For this review, take the finished solid that the model builds, in its own axes (mm). Face numbers are marked on the shaded views. Coordinates: 2 decimals unless noted, no trailing zeros. Loops run counter-clockwise (first coordinate to the right, second up) from the corner with the lowest first, then second, coordinate; pieces in that order, holes last. Notation, with made-up numbers: M 58,56 L 108,56 A16 cw 108,85 Z; hole C 73,63 d5. An arc over 180 degrees is marked long. Put each result on its own line as item: value.
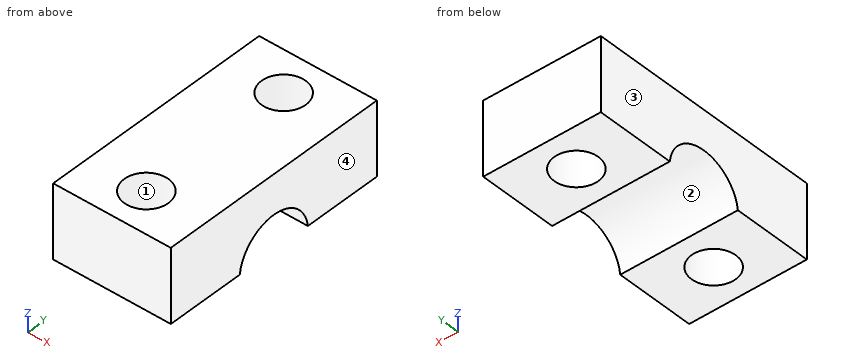
```python
from build123d import *

# Parameters (mm, degrees)
BOSS_EXTRUDE1_DEPTH = 12
SKETCH2_R           = 2.25
CUT_EXTRUDE1_DEPTH  = 19.761663039
SKETCH3_W           = 12
SKETCH3_H           = 24
CUT_EXTRUDE2_DEPTH  = 0.5


with BuildPart() as part:
    # Sketch1 → Boss-Extrude1 (new body)
    with BuildSketch(Plane(origin=(0, 0, 0), x_dir=(0, 0, -1), z_dir=(1, 0, 0))):
        with BuildLine():
            Line((8, -4), (8, -12))
            Line((8, -12), (0, -12))
            Line((0, -12), (0, 12))
            Line((0, 12), (8, 12))
            Line((8, 12), (8, 4))
            ThreePointArc((8, 4), (4, 0), (8, -4))
        make_face()
    extrude(amount=BOSS_EXTRUDE1_DEPTH)

    # Sketch2 → Cut-Extrude1 (cut, through all)
    with BuildSketch(Plane.XY):
        with Locations((6, 8)):
            Circle(SKETCH2_R)
        with Locations((6, -8)):
            Circle(SKETCH2_R)
    extrude(amount=-CUT_EXTRUDE1_DEPTH, mode=Mode.SUBTRACT)

    # Sketch3 → Cut-Extrude2 (cut)
    with BuildSketch(Plane(origin=(0, 0, -8), x_dir=(-1, 0, 0), z_dir=(0, 0, -1))):
        with Locations((-6, 0)):
            Rectangle(SKETCH3_W, SKETCH3_H)
    extrude(amount=-CUT_EXTRUDE2_DEPTH, mode=Mode.SUBTRACT)


solid = part.part
```
(1) Add section A-A (y = 8). Write out the cut boundary in (x, z), plus the area to 4 significant figures.
Determined:
outline: M 0,-7.5 L 3.75,-7.5 L 3.75,0 L 0,0 Z; M 8.25,-7.5 L 12,-7.5 L 12,0 L 8.25,0 Z
area: 56.25 mm^2
(2) Draft analysis for pull direction X (two halves, no side actions). For the marked faces 1, 2, 3 and 4, state which applies: +X half, -X half, draft (parallel to the pull), parting line (faces both ways), or undercut.
Determined:
face 1: undercut
face 2: draft
face 3: -X half
face 4: +X half
(3) Add section B-B (z = -6). Write out the cut boundary in (x, y), plus the area to 3 significant figures.
Determined:
outline: M 0,-12 L 12,-12 L 12,-3.46 L 0,-3.46 Z; M 0,3.46 L 12,3.46 L 12,12 L 0,12 Z; hole C 6,-8 d4.5; hole C 6,8 d4.5
area: 173 mm^2
(4) Add section D-D (z = -1.5). Write out the cut boundary in (x, y).
Determined:
outline: M 0,-12 L 12,-12 L 12,12 L 0,12 Z; hole C 6,-8 d4.5; hole C 6,8 d4.5
(5) Add section C-C (x = 6). Write out the cut boundary in (y, z).
Determined:
outline: M -12,-7.5 L -10.25,-7.5 L -10.25,0 L -12,0 Z; M -5.75,-7.5 L -3.97,-7.5 A4 cw 3.97,-7.5 L 5.75,-7.5 L 5.75,0 L -5.75,0 Z; M 10.25,-7.5 L 12,-7.5 L 12,0 L 10.25,0 Z
(6) Wall thickness on line 1 along Y through (x, z) = (6, -1.75); line 2 along Y through (x, z) = (4.75, -0.5); line 3 along Y through (x, z) = (6, -5.5): over which ranges is each line inside the solid? List them lowest first. Write a range as [from, to].
Determined:
line 1: y = [-12, -10.25], [-5.75, 5.75], [10.25, 12]
line 2: y = [-12, -9.87], [-6.13, 6.13], [9.87, 12]
line 3: y = [-12, -10.25], [-5.75, -3.12], [3.12, 5.75], [10.25, 12]
